```python
from build123d import *

# Parameters (mm, degrees)
BOX008_W      = 5
BOX008_H      = 10
BOX008_DEPTH  = 5
BOX007_W      = 5
BOX007_H      = 5
BOX007_DEPTH  = 10
TUBE003_R     = 5
TUBE003_R_2   = 3
TUBE003_DEPTH = 5


with BuildPart() as cube008:
    # Box008 → Box008 (new body)
    with BuildSketch(Plane(origin=(0, -2, 3), x_dir=(1, 0, 0), z_dir=(0, 0, 1))):
        with Locations((2.5, 5)):
            Rectangle(BOX008_W, BOX008_H)
    extrude(amount=BOX008_DEPTH)


with BuildPart() as cube007:
    # Box007 → Box007 (new body)
    with BuildSketch(Plane(origin=(0, 3, -2), x_dir=(1, 0, 0), z_dir=(0, 0, 1))):
        with Locations((2.5, 2.5)):
            Rectangle(BOX007_W, BOX007_H)
    extrude(amount=BOX007_DEPTH)


with BuildPart() as cut007:
    # Tube003 → Tube003 (new body)
    with BuildSketch(Plane(origin=(0, 3, 3), x_dir=(0, 0, -1), z_dir=(1, 0, 0))):
        Circle(TUBE003_R)
        Circle(TUBE003_R_2, mode=Mode.SUBTRACT)
    extrude(amount=TUBE003_DEPTH)

    # Cut006: cut Cube007
    add(cube007.part, mode=Mode.SUBTRACT)

    # Cut007: cut Cube008
    add(cube008.part, mode=Mode.SUBTRACT)


solid = cut007.part
```
The model under review builds one solid part; all positions refer to its coordinate system, in mm. Give positions to 0.01 mm unless a question says otherwise; leave off trailing zeros. Write each loop counter-clockwise with the first axis right and the second up, starting at its lowest first coordinate (ties: lowest second). Pieces come first, ordered by that corner, then holes. Notation, with made-up numbers: M -35,77.25 L 5,77.25 A12 ccw 5,83.25 Z; hole C -26,64.5 d4. An arc over 180 degrees is marked long. Answer in a Markdown table with one row per item.
Item 1: For P1, Ø2, axis at x = 4, y = 1, coming from the -Z side, flat-tipped, find the tip position at first contact; note if it passes through.
Check sheet entries:
| item | result |
|---|---|
| P1 | z = -1.9 |
Item 2: Add section A-A on x = 4. Give the boundary of the cut face in (y, z).
Check sheet entries:
| item | result |
|---|---|
| outline | M -2,3 A5 ccw 3,-2 L 3,0 A3 cw 0,3 Z |
Item 3: Add section B-B on z = 0.75. Give the boundary of the cut face in (x, y), plus the area to 3 significant figures.
Check sheet entries:
| item | result |
|---|---|
| outline | M 0,-1.47 L 5,-1.47 L 5,1.02 L 0,1.02 Z |
| area | 12.4 mm2 |
Item 4: For line 1 along Z through (x, y) = (3.85, -1); line 2 along Y through (x, z) = (0.75, 0.5); line 3 along Y through (x, z) = (1.75, 1.6), list the stretches that pass through material, from the lowest coordinate up.
Check sheet entries:
| item | result |
|---|---|
| line 1 | 0 to 3 |
| line 2 | -1.33 to 1.34 |
| line 3 | -1.8 to 0.35 |
